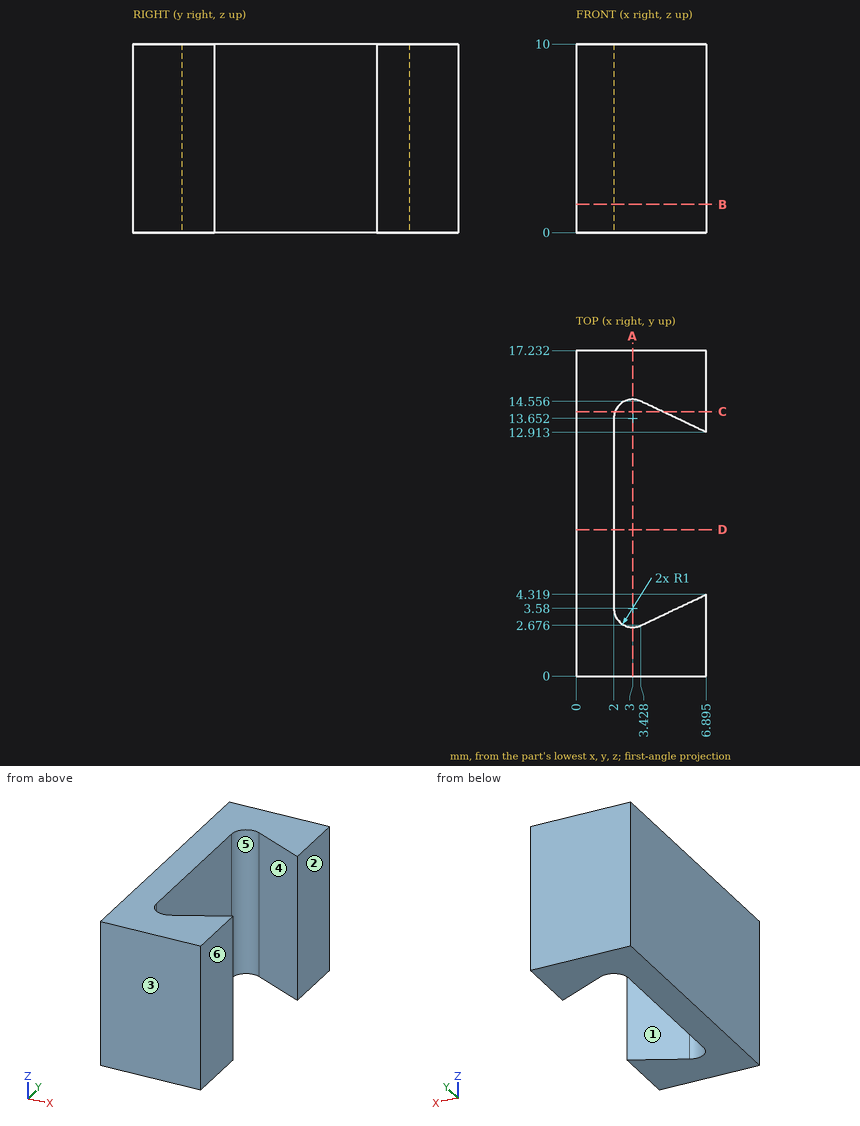
Geometry check sheet. Reference: drawing and pictorial views, mm from the part's lowest x, y, z. A direction names the side the tool comes from. Coordinates: 2 decimals unless noted, no trailing zeros. Loops run counter-clockwise (first coordinate to the right, second up) from the corner with the lowest first, then second, coordinate; pieces in that order, holes last. Notation, with made-up numbers: M 27.5,75 L 58.5,75 A29 ccw 58.5,97 Z; hole C 70,-4 d3. An arc over 180 degrees is marked long. One line per item, written item: value.
1. Material ranges on line 1 along Y through (x, z) = (5.25, 6.5); line 2 along Y through (x, z) = (4.75, 3); line 3 along X through (y, z) = (10.5, 1.5), recorded low to high. Write a range as from..to.
Answers follow:
line 1: 0..3.54, 13.69..17.23
line 2: 0..3.3, 13.93..17.23
line 3: 0..2
2. Section check C-C on y = 14. Record the cut outline in (x, z) (1 decimal).
Answers follow:
outline: M 0,0 L 2.1,0 L 2.1,10 L 0,10 Z; M 4.6,0 L 6.9,0 L 6.9,10 L 4.6,10 Z
3. Section check B-B on z = 1.5. Record the cut outline in (x, y) (1 decimal).
Answers follow:
outline: M 0,0 L 6.9,0 L 6.9,4.3 L 3.4,2.7 A1 cw 2,3.6 L 2,13.7 A1 cw 3.4,14.6 L 6.9,12.9 L 6.9,17.2 L 0,17.2 Z
4. Gauge pin test, flat ends, axial feed: P1, Ø1.5, axis at x = 5.5, z = 6, coming from the -Y side; P2, Ø2, axis at y = 8.5, z = 5.5, coming from the +X side. Record the tip position at first contact, or that the pin passes through.
Answers follow:
P1: y = 0
P2: x = 2
5. Set-up check for the marked faces 5 and 6: record each of +Z, -Z, +X, -X, +Y, -Y from which the full face is reachable in a straight line by a thin tool's end or side.
Answers follow:
face 5: +Z, -Z
face 6: +Z, -Z, +X, +Y, -Y
6. Mould release check, pull along Y, two halves, no side actions. Record for the marked faces 1, 2, 3 and 4: pulls with the +Y half, pulls with the -Y half, needs draft (parallel to the pull), parting line crosses it, or undercut.
Answers follow:
face 1: undercut
face 2: needs draft
face 3: pulls with the -Y half
face 4: undercut
7. Section check A-A on x = 3. Record the cut outline in (y, z).
Answers follow:
outline: M 0,0 L 2.58,0 L 2.58,10 L 0,10 Z; M 14.65,0 L 17.23,0 L 17.23,10 L 14.65,10 Z
8. Section check D-D on y = 7.75. Record the cut outline in (x, z), plus the area to 3 significant figures.
Answers follow:
outline: M 0,0 L 2,0 L 2,10 L 0,10 Z
area: 20.0 mm^2
